Here's how the part is built. I have some questions about the finished solid (model axes, mm). Face numbers are marked on the shaded views. Coordinates: 2 decimals unless noted, no trailing zeros.
```python
from build123d import *

# Parameters (mm, degrees)
SKETCH1_R                = 75
BASE_EXTRUDE_DEPTH       = 32
SHELL1_T                 = -6
SKETCH4_R                = 42.5
CUT_EXTRUDE2_DEPTH       = 110.206226929
BOSS_EXTRUDE1_START      = -6
BOSS_EXTRUDE1_DEPTH      = 6
CUT_EXTRUDE1_REACH       = 112.788
SKETCH3_R                = 6
FILLET1_R                = 3
CIRPATTERN1_COUNT        = 4
FILLET1_OF_CIRPATTERN1_R = 3
SKETCH5_R                = 6
CUT_EXTRUDE3_DEPTH       = 110.206226929
CIRPATTERN2_COUNT        = 8
FILLET2_R                = 2


with BuildPart() as part:
    # Sketch1 → Base-Extrude (new body)
    with BuildSketch(Plane(origin=(0, 0, 0), x_dir=(1, 0, 0), z_dir=(0, 1, 0))):
        with Locations(Location((0, 0, 0), (0, 0, 270))):
            Circle(SKETCH1_R)
    extrude(amount=BASE_EXTRUDE_DEPTH)

    # Shell1
    shell1_openings = [part.faces().sort_by_distance(p)[0] for p in [
        (0, 32, 0),
    ]]
    offset(amount=SHELL1_T, openings=shell1_openings, kind=Kind.INTERSECTION)

    # Sketch4 → Cut-Extrude2 (cut, through all)
    with BuildSketch(Plane(origin=(0, 6, 0), x_dir=(-1, 0, 0), z_dir=(0, 1, 0))):
        with Locations(Location((0, 0, 0), (0, 0, 90))):
            Circle(SKETCH4_R)
    extrude(amount=-CUT_EXTRUDE2_DEPTH, mode=Mode.SUBTRACT)

    # Sketch2 → Boss-Extrude1 (add)
    with BuildSketch(Plane(origin=(0, 32, 0), x_dir=(-1, 0, 0), z_dir=(0, 1, 0)).offset(BOSS_EXTRUDE1_START)):
        with BuildLine():
            Line((-10, -68.271516755), (-10, -60))
            ThreePointArc((-10, -60), (0, -50), (10, -60))
            Line((10, -60), (10, -68.271516755))
            ThreePointArc((10, -68.271516755), (0, -69), (-10, -68.271516755))
        make_face()
    boss_extrude1 = extrude(amount=BOSS_EXTRUDE1_DEPTH)

    # Sketch3 → Cut-Extrude1 (cut, up to next)
    with BuildSketch(Plane(origin=(0, 32, 0), x_dir=(-1, 0, 0), z_dir=(0, 1, 0)), mode=Mode.PRIVATE) as cut_extrude1_sk1:
        with Locations(Location((0, -60, 0), (0, 0, 90))):
            Circle(SKETCH3_R)
    cut_extrude1_tool1 = extrude(cut_extrude1_sk1.sketch, amount=-CUT_EXTRUDE1_REACH, mode=Mode.PRIVATE) & part.part
    cut_extrude1 = cut_extrude1_tool1.solids().sort_by_distance((0, 32, -60))[0]
    add(cut_extrude1, mode=Mode.SUBTRACT)

    # Fillet1
    fillet1_edges = [part.edges().sort_by_distance(p)[0] for p in [
        (-10, 29, -68.271516755),
        (10, 29, -68.271516755),
    ]]
    fillet(fillet1_edges, radius=FILLET1_R)

    # CirPattern1: Boss-Extrude1, Cut-Extrude1 ×4 about axis
    cirpattern1_axis = Axis((0, 0, 0), (0, 1, 0))
    add([boss_extrude1.rotate(cirpattern1_axis, i * 360 / CIRPATTERN1_COUNT) for i in range(1, CIRPATTERN1_COUNT)])
    add([cut_extrude1.rotate(cirpattern1_axis, i * 360 / CIRPATTERN1_COUNT) for i in range(1, CIRPATTERN1_COUNT)], mode=Mode.SUBTRACT)

    # Fillet1 of CirPattern1
    fillet1_of_cirpattern1_edges = [part.edges().sort_by_distance(p)[0] for p in [
        (-68.271516755, 29, 10),
        (-68.271516755, 29, -10),
        (10, 29, 68.271516755),
        (-10, 29, 68.271516755),
        (68.271516755, 29, -10),
        (68.271516755, 29, 10),
    ]]
    fillet(fillet1_of_cirpattern1_edges, radius=FILLET1_OF_CIRPATTERN1_R)

    # Sketch5 → Cut-Extrude3 (cut, through all)
    with BuildSketch(Plane(origin=(0, 6, 0), x_dir=(-1, 0, 0), z_dir=(0, 1, 0))):
        with Locations(Location((0, -60, 0), (0, 0, 90))):
            Circle(SKETCH5_R)
    cut_extrude3 = extrude(amount=-CUT_EXTRUDE3_DEPTH, mode=Mode.SUBTRACT)

    # CirPattern2: Cut-Extrude3 ×8 about axis
    cirpattern2_axis = Axis((0, 0, 0), (0, 1, 0))
    for i in range(1, CIRPATTERN2_COUNT):
        add(cut_extrude3.rotate(cirpattern2_axis, i * 360 / CIRPATTERN2_COUNT), mode=Mode.SUBTRACT)

    # Fillet2
    fillet2_edges = [part.edges().sort_by_distance(p)[0] for p in [
        (0, 6, -69),
        (0, 6, -42.5),
    ]]
    fillet(fillet2_edges, radius=FILLET2_R)


solid = part.part
```
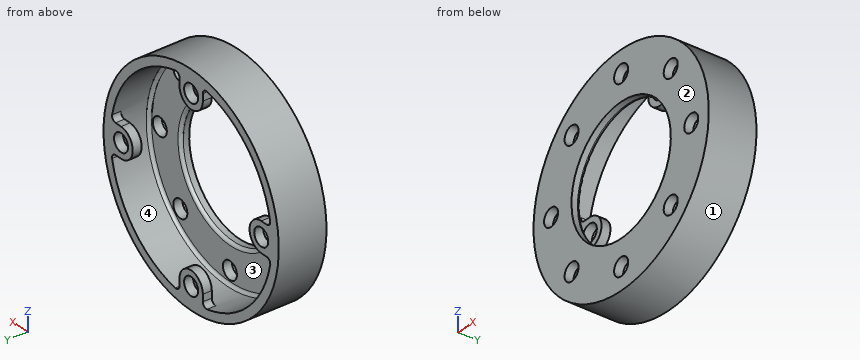
1) Will these pins go through, and if not, where does the flat tip stop? pin 1 (2 mm diameter, centred on y = 16, z = 45.5, fed in from +X); pin 2 (6 mm diameter, centred on x = 39, y = 8.5, fed in from -Z); pin 3 (5.5 mm diameter, centred on x = -3.5, z = 55, fed in from -Y); pin 4 (15.5 mm diameter, centred on x = 42.43, z = -42.43, fed in from +Y).
Values follow:
pin 1: stops at x = 60.37
pin 2: stops at z = -65.8
pin 3: stops at y = 0
pin 4: stops at y = 6.15
2) We'd pull the mould along X, two halves only. Please class the marked faces 1, 2, 3 and 4: pulls with the +X half, pulls with the -X half, needs draft (parallel to the pull), parting line crosses it, or undercut.
Values follow:
face 1: parting line crosses it
face 2: needs draft
face 3: undercut
face 4: undercut
3) I need wall thicknesses on probe 1 along Y at (x, z) = (-59.5, 7); probe 2 along Z at (x, y) = (60, 29); probe 3 along X at (y, z) = (18, 0). Which ranges of each line are inside material? Lowest first, please.
Values follow:
probe 1: y = 0 to 6, 26 to 32
probe 2: z = -45 to -34.07, -10 to -6, 6 to 10, 34.07 to 45
probe 3: x = -75 to -69, 69 to 75
4) Imagine slicing it at A-A on y = 29.5. Count the separate pieces of the cut face and the enclosed holes in it, then the cut area to 3 significant figures.
Values follow:
separate pieces: 1
enclosed holes: 5
area: 3,610 mm2
